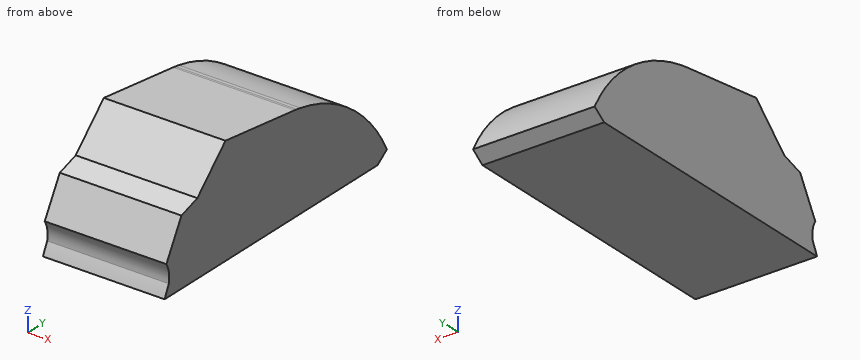
from build123d import *

# Parameters (mm, degrees)
F1_DEPTH      = 15.24
F1_DEPTH_BACK = 15.24


with BuildPart() as f1:
    # F0 (on Right) → F1 (new body, two sides)
    with BuildSketch(Plane.YZ) as f1_sk:
        with BuildLine():
            ThreePointArc((-1.434684, 2.266193), (-13.407881, 16.531469), (-30.440374, 24.064712))
            ThreePointArc((-30.440374, 24.064712), (-21.972596, 20.363563), (-15.764277, 13.518233))
            ThreePointArc((-15.764277, 13.518233), (-15.114308, 11.234153), (-16.148772, 9.096545))
            Line((-16.148772, 9.096545), (-50.502049, 12.267617))
            ThreePointArc((-50.502049, 12.267617), (-55.179249, 9.077793), (-57.481937, 3.905869))
            Line((-57.481937, 3.905869), (-4.613936, 0))
            Line((-4.613936, 0), (-1.434684, 2.266193))
        make_face()
        with BuildLine():
            ThreePointArc((-30.440374, 24.064712), (-31.030504, 24.176615), (-31.623462, 24.272407))
            ThreePointArc((-31.623462, 24.272407), (-31.031161, 24.172873), (-30.440374, 24.064712))
        make_face()
        with BuildLine():
            ThreePointArc((-74.524937, 2.932697), (-75.260293, 1.480311), (-75.937681, 0))
            ThreePointArc((-75.937681, 0), (-75.049977, 1.378997), (-74.524937, 2.932697))
        make_face()
        Polygon((-4.613936, 0), (-57.481937, 3.905869), (-60.1734, 0), align=None)
        with BuildLine():
            ThreePointArc((-50.502049, 12.267617), (-42.703408, 20.296684), (-32.278686, 24.372209))
            Line((-32.278686, 24.372209), (-55.559464, 27.360039))
            Line((-55.559464, 27.360039), (-64.979583, 18.324416))
            ThreePointArc((-64.979583, 18.324416), (-58.204998, 14.186486), (-50.502049, 12.267617))
        make_face()
        with BuildLine():
            ThreePointArc((-30.440374, 24.064712), (-31.031161, 24.172873), (-31.623462, 24.272407))
            ThreePointArc((-31.623462, 24.272407), (-31.950873, 24.323626), (-32.278686, 24.372209))
            ThreePointArc((-32.278686, 24.372209), (-42.703408, 20.296684), (-50.502049, 12.267617))
            Line((-50.502049, 12.267617), (-16.148772, 9.096545))
            ThreePointArc((-16.148772, 9.096545), (-15.114308, 11.234153), (-15.764277, 13.518233))
            ThreePointArc((-15.764277, 13.518233), (-21.972596, 20.363563), (-30.440374, 24.064712))
        make_face()
        with BuildLine():
            ThreePointArc((-57.481937, 3.905869), (-55.179249, 9.077793), (-50.502049, 12.267617))
            ThreePointArc((-50.502049, 12.267617), (-58.204998, 14.186486), (-64.979583, 18.324416))
            Line((-64.979583, 18.324416), (-70.306638, 16.641369))
            Line((-70.306638, 16.641369), (-75.360931, 7.750814))
            ThreePointArc((-75.360931, 7.750814), (-74.486311, 5.420985), (-74.524937, 2.932697))
            ThreePointArc((-74.524937, 2.932697), (-75.049977, 1.378997), (-75.937681, 0))
            Line((-75.937681, 0), (-60.1734, 0))
            Line((-60.1734, 0), (-57.481937, 3.905869))
        make_face()
    extrude(amount=F1_DEPTH)
    extrude(f1_sk.sketch, amount=-F1_DEPTH_BACK)


solid = f1.part
Read the model definition and answer for the solid it produces. Units are mm, in the model's axes. Coordinates: 2 decimals unless noted, no trailing zeros. Order: outer loops, then holes, each group sorted by start corner. A loop starts at its lowest first (then second) coordinate and runs counter-clockwise, first axis right, second up. Notation, with made-up numbers: (-13, 80) - (30, 80) arc R11 ccw to (30, 92) - close; hole circle Ø1 at (-17, 54.5). An arc over 180 degrees is marked (long way). Use one line per item in the form item = value.
(1) Straight lines are drawn through the part: L1, parallel to Z at x = -14, y = -59; L2, parallel to Z at x = -8, y = -68; L3, parallel to Y at x = -4, z = 11.5. For each, find the intervals that lie inside material, in ascending order.
Computed values:
L1 = 0 to 24.06
L2 = 0 to 17.37
L3 = -73.23 to -7.85
(2) Section A-A, the plane x = 9.5 is taken. Give the vertices of the cut face in (y, z), then the cut area to 3 significant figures.
Computed values:
outline = (-75.94, 0) - (-4.61, 0) - (-1.43, 2.27) arc R41.19 ccw to (-30.44, 24.06) arc R22.06 ccw to (-31.62, 24.27) arc R41.19 ccw to (-32.28, 24.37) - (-55.56, 27.36) - (-64.98, 18.32) - (-70.31, 16.64) - (-75.36, 7.75) arc R6.68 cw to (-74.52, 2.93) arc R41.19 ccw to start
area = 1,490 mm²
(3) Given pin 1 Ø4 at (x, y) = (-8.5, -50.5) entering from +Z; pin 2 Ø5 at (x, z) = (1, 24) entering from -Y, each flat-ended and moving along its own axis, determine where each tip first touches the part or whether it passes through.
Computed values:
pin_1 = 26.97
pin_2 = -61.67
(4) Section C-C, the plane y = -69.5 is taken. Give the vertices of the cut face in (x, z), then the cut area to 3 significant figures.
Computed values:
outline = (-15.24, 0) - (15.24, 0) - (15.24, 16.9) - (-15.24, 16.9) - close
area = 515 mm²
(5) Section B-B, the plane z = 6.5 is taken. Give the vertices of the cut face in (x, y), then the cut area to 3 significant figures.
Computed values:
outline = (-15.24, -74.77) - (15.24, -74.77) - (15.24, -3.91) - (-15.24, -3.91) - close
area = 2,160 mm²
